Can you work these out from the model? Positions are in its coordinate system, mm. Coordinates: 2 decimals unless noted, no trailing zeros. Order: outer loops, then holes, each group sorted by start corner. A loop starts at its lowest first (then second) coordinate and runs counter-clockwise, first axis right, second up.
```python
from build123d import *

# Parameters (mm, degrees)
PAD013_DEPTH        = 3
HOLE012_D           = 3.4
HOLE012_DEPTH       = 25
HOLE012_CSINK_D     = 6.1
HOLE012_CSINK_ANGLE = 90


with BuildPart() as body020:
    # Sketch042 (on Face1 of Binder029) → Pad013 (new body)
    with BuildSketch(Plane.XY):
        Polygon((-18.5, -59.5), (-15.952208, -66.5), (-3.047792, -66.5), (-0.5, -59.5), align=None)
    extrude(amount=PAD013_DEPTH)

    # Hole012
    with Locations(Plane(origin=(0, 0, 0), x_dir=(1, 0, 0), z_dir=(0, 0, -1))):
        with Locations((-9.5, 63)):
            CounterSinkHole(HOLE012_D / 2, HOLE012_CSINK_D / 2, depth=HOLE012_DEPTH, counter_sink_angle=HOLE012_CSINK_ANGLE)


with BuildPart() as part_mirroring:
    # Part__Mirroring: instance of Body020
    add(body020.part.mirror(Plane(origin=(0, 0, 0), x_dir=(1, 0, 0), z_dir=(0, 1, 0))))


solid = part_mirroring.part
```
1. Please list where these lines run through material, in increasing order: probe 1 along Y at (x, z) = (-9.5, 2.15); probe 2 along X at (y, z) = (63, 2); probe 3 along X at (y, z) = (64.5, 2.3).
Completed:
probe 1: y = 59.5 to 61.3, 64.7 to 66.5
probe 2: x = -17.23 to -11.2, -7.8 to -1.77
probe 3: x = -16.68 to -10.3, -8.7 to -2.32
2. I'm going to push a flat-ended pin straight in: pin 1 (3 mm diameter, centred on x = -9.5, y = 63, fed in from +Z). Where does the tip first touch, or does it pass through?
Completed:
pin 1: passes through
3. Imagine slicing it at C-C on z = 1.85. Please give me the cut outline in (x, y), then the cut area to 3 significant figures.
Completed:
outline: (-18.5, 59.5) - (-0.5, 59.5) - (-3.05, 66.5) - (-15.95, 66.5) - close; hole circle Ø3.4 at (-9.5, 63)
area: 99.1 mm2
4. Thinking about a two-plate mould opening in X: for faces 1 (the flat face through (-10, 66.5, 1)), 2 (the cylindrical face through (-9.279, 64.686, 2.187)), 3 (the flat face through (-1.79, 63.05, 1.48)), which applies, pulls with the +X half, pulls with the -X half, needs draft (parallel to the pull), parting line crosses it, or undercut?
Completed:
face 1: needs draft
face 2: undercut
face 3: pulls with the +X half
5. Imagine slicing it at A-A on x = -9.5. Please give me the cut outline in (y, z), then the cut area to 3 significant figures.
Completed:
outline: (59.5, 0) - (59.95, 0) - (61.3, 1.35) - (61.3, 3) - (59.5, 3) - close; (64.7, 1.35) - (66.05, 0) - (66.5, 0) - (66.5, 3) - (64.7, 3) - close
area: 8.98 mm2
6. Imagine slicing it at B-B on y = 63. Please give me the cut outline in (x, z), then the cut area to 3 significant figures.
Completed:
outline: (-17.23, 0) - (-12.55, 0) - (-11.2, 1.35) - (-11.2, 3) - (-17.23, 3) - close; (-7.8, 1.35) - (-6.45, 0) - (-1.77, 0) - (-1.77, 3) - (-7.8, 3) - close
area: 34.3 mm2
